Design review of the part built by this model. Coordinates are the model's own, in mm. Face numbers are marked on the shaded views. A direction names the side the tool comes from. Give positions to 0.01 mm unless a question says otherwise; leave off trailing zeros. Loops run counter-clockwise (first coordinate to the right, second up) from the corner with the lowest first, then second, coordinate; pieces in that order, holes last.
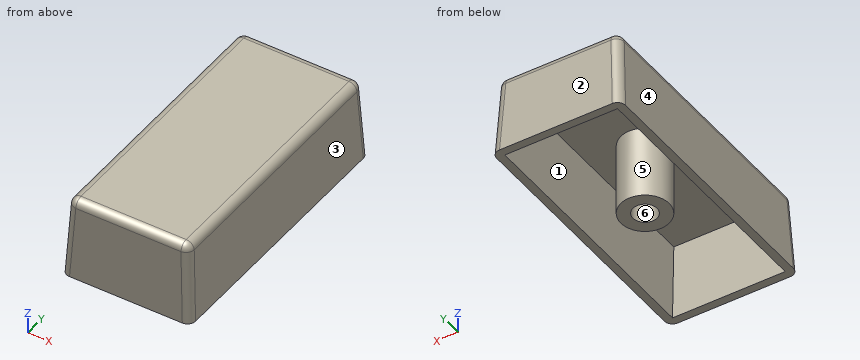
from build123d import *

# Parameters (mm, degrees)
ESQUISSE1_W        = 16
ESQUISSE1_H        = 34
BOSS_EXTRU_1_DEPTH = 10
BOSS_EXTRU_1_TAPER = 3
CONG_1_R           = 1
COQUE1_OUTLINE_W   = 13.05391528
COQUE1_OUTLINE_H   = 31.05391528
COQUE1_DEPTH       = 9
COQUE1_DRAFT       = 3
ESQUISSE2_R        = 3
ESQUISSE2_R_2      = 1.5
BOSS_EXTRU_2_DEPTH = 9


# Read off the part's stored shape, not the designer's step: Coque1
with BuildPart() as part:
    # Esquisse1 → Boss.-Extru.1 (new body)
    with BuildSketch(Plane.XY):
        Rectangle(ESQUISSE1_W, ESQUISSE1_H)
    extrude(amount=BOSS_EXTRU_1_DEPTH, taper=BOSS_EXTRU_1_TAPER)

    # Congé1
    cong_1_edges = [part.edges().sort_by_distance(p)[0] for p in [
        (7.475922207, 0, 10),
        (0, 16.475922207, 10),
        (-7.475922207, 0, 10),
        (-7.737960642, 16.737960642, 5.000008814),
        (7.737961104, 16.737961104, 5),
        (7.737960642, -16.737960642, 5.000008814),
        (-7.737961104, -16.737961104, 5),
        (0, -16.475922207, 10),
    ]]
    fillet(cong_1_edges, radius=CONG_1_R)


with BuildPart() as coque1_tool:
    # Coque1 outline → Coque1 (with draft: the straight prism first)
    with BuildSketch(Plane.XY.offset(9)):
        Rectangle(COQUE1_OUTLINE_W, COQUE1_OUTLINE_H)
    extrude(amount=-COQUE1_DEPTH)
    # Coque1: the draft: its side faces are tilted about the plane it starts from
    coque1_sides = [coque1_tool.faces().sort_by_distance(p)[0] for p in [
        (-6.52695764, 0, 4.5),
        (0, -15.52695764, 4.5),
        (6.52695764, 0, 4.5),
        (0, 15.52695764, 4.5),
    ]]
    draft(coque1_sides, Plane.XY.offset(9), COQUE1_DRAFT)


with BuildPart() as part_1:
    add(part.part)

    # Coque1: cut by coque1_tool
    add(coque1_tool.part, mode=Mode.SUBTRACT)

    # Esquisse2 → Boss.-Extru.2 (add)
    with BuildSketch(Plane(origin=(0, 0, 9), x_dir=(-1, 0, 0), z_dir=(0, 0, -1))):
        with Locations(Location((0, 0, 0), (0, 0, 180))):
            Circle(ESQUISSE2_R)
        with Locations(Location((0, 0, 0), (0, 0, 180))):
            Circle(ESQUISSE2_R_2, mode=Mode.SUBTRACT)
    extrude(amount=BOSS_EXTRU_2_DEPTH)


solid = part_1.part
Q1. Take a section at B-B (y = 14). Give the boundary of the cut face in (x, z).
Results:
outline: (-8, 0) - (-7, 0) - (-6.53, 9) - (6.53, 9) - (7, 0) - (8, 0) - (7.53, 9.05) arc R1 ccw to (6.53, 10) - (-6.53, 10) arc R1 ccw to (-7.53, 9.05) - close
Q2. Take a section at D-D (y = 0). Give the boundary of the cut face in (x, z), plus the area to 3 significant figures.
Results:
outline: (-8, 0) - (-7, 0) - (-6.53, 9) - (-3, 9) - (-3, 0) - (-1.5, 0) - (-1.5, 9) - (1.5, 9) - (1.5, 0) - (3, 0) - (3, 9) - (6.53, 9) - (7, 0) - (8, 0) - (7.53, 9.05) arc R1 ccw to (6.53, 10) - (-6.53, 10) arc R1 ccw to (-7.53, 9.05) - close
area: 59.6 mm2
Q3. Wall thickness on line 1 (Y direction, x = -2.75, z = 4.5); line 2 (Y direction, x = 0.25, z = 8.75); line 3 (Z direction, x = 4, y = 11.5): over which ranges is each line inside the solid? List them lowest first.
Results:
line 1: y = -16.76 to -15.76, -1.2 to 1.2, 15.76 to 16.76
line 2: y = -16.54 to -15.54, -2.99 to -1.48, 1.48 to 2.99, 15.54 to 16.54
line 3: z = 9 to 10
Q4. Tool access review of the marked faces 1 and 2: name each direction out of +Z, -Z, +X, -X, +Y, -Y from which nothing blocks a thin tool from reaching the whole face with its end or side.
Results:
face 1: -Z
face 2: +Z, +X, -X, +Y
Q5. Draft analysis for pull direction X (two halves, no side actions). For the marked faces 3, 4, 5 and 6, state which applies: pulls with the +X half, pulls with the -X half, needs draft (parallel to the pull), parting line crosses it, or undercut.
Results:
face 3: pulls with the +X half
face 4: pulls with the -X half
face 5: undercut
face 6: undercut
Q6. Take a section at C-C (z = 5.25). Give the number of separate pieces and of enclosed holes in the cut face, plus the area to 3 significant figures.
Results:
separate pieces: 2
enclosed holes: 2
area: 114 mm2
Q7. Insertion check: pin 1 (1.5 mm diameter, centred on x = 3.5, y = -4.5, fed in from -Z); pin 2 (1 mm diameter, centred on x = -5, z = 3, fed in from +Y); pin 3 (3 mm diameter, centred on x = -0.5, z = 5, fed in from -Y). Each pin has a flat end and moves straight along its axis. Give the tip position at first contact, or say it passes through.
Results:
pin 1: stops at z = 9
pin 2: stops at y = 16.87
pin 3: stops at y = -16.82
Q8. Take a section at A-A (x = 0). Give the boundary of the cut face in (y, z).
Results:
outline: (-17, 0) - (-16, 0) - (-15.53, 9) - (-3, 9) - (-3, 0) - (-1.5, 0) - (-1.5, 9) - (1.5, 9) - (1.5, 0) - (3, 0) - (3, 9) - (15.53, 9) - (16, 0) - (17, 0) - (16.53, 9.05) arc R1 ccw to (15.53, 10) - (-15.53, 10) arc R1 ccw to (-16.53, 9.05) - close
